Autodesk Inventor part; units mm, degrees
ref_plane "YZ Plane" through (0, 0, 0) normal (1, 0, 0) x (0, 1, 0)
ref_plane "XZ Plane" through (0, 0, 0) normal (0, 1, 0) x (-1, 0, 0)
ref_plane "XY Plane" through (0, 0, 0) normal (0, 0, 1) x (1, 0, 0)
sketch "Sketch1" plane through (0, 0, 0) normal (0, 1, 0) x (-1, 0, 0)
  line L0 (0, 0) -> (406.4, 0)
  line L1 (406.4, 0) -> (406.4, -1219.2)
  line L2 (406.4, -1219.2) -> (0, -1219.2)
  line L3 (0, -1219.2) -> (0, 0)
  line L4 (0, -609.6) -> (101.6, -609.6)
  line L5 (101.6, -609.6) -> (184.15, -609.6)
  line L6 (184.15, -609.6) -> (273.05, -609.6)
  line L7 (349.25, -533.4) -> (196.85, -533.4)
  line L8 (196.85, -533.4) -> (196.85, -685.8)
  line L9 (196.85, -685.8) -> (349.25, -685.8)
  line L10 (349.25, -685.8) -> (349.25, -533.4)
  line L11 (349.25, -533.4) -> (196.85, -685.8) construction
  line L12 (196.85, -533.4) -> (349.25, -685.8) construction
  dimension "d0" = 1219.2
  dimension "d1" = 406.4
  dimension "d2" = 101.6
  dimension "d3" = 82.55
  dimension "d4" = 88.9
  dimension "d5" = 152.4
  dimension "d6" = 152.4
extrude "Extrusion1" add sketch "Sketch1" along normal blind 12.7
properties part number "backBoard" material "Wood (Birch)"
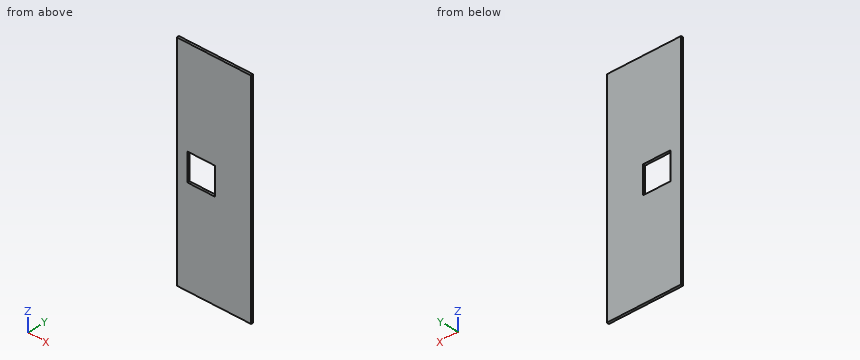
Model file for the job. Use its own axes, mm. Give positions to 0.01 mm unless a question says otherwise; leave off trailing zeros. Loops run counter-clockwise (first coordinate to the right, second up) from the corner with the lowest first, then second, coordinate; pieces in that order, holes last.
1) Saw through at B-B (y = 10.5). Write the cut outline in (x, z).
2) Saw through at A-A (x = -241.5). Write the cut outline in (y, z).
3) Wall check: line 1 (Z direction, x = -330.5, y = 4); line 2 (X direction, y = 6.5, z = -565). Give the ranges that are in metal, low to high.
4) Flat gauge pin, fed straight in: pin 1 Ø3 at (x, y) = (-77.5, 7) entering from +Z. Where does the tip first touch, or does it go through?
Answer block:
1. outline: (-406.4, -1219.2) - (0, -1219.2) - (0, 0) - (-406.4, 0) - close; hole (-349.25, -685.8) - (-196.85, -685.8) - (-196.85, -533.4) - (-349.25, -533.4) - close
2. outline: (0, -1219.2) - (12.7, -1219.2) - (12.7, -685.8) - (0, -685.8) - close; (0, -533.4) - (12.7, -533.4) - (12.7, 0) - (0, 0) - close
3. line 1: z = -1219.2 to -685.8, -533.4 to 0
3. line 2: x = -406.4 to -349.25, -196.85 to 0
4. pin 1: stops at z = 0
